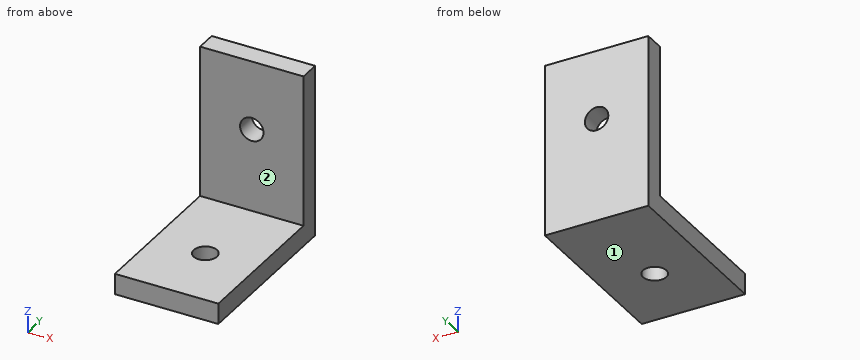
```python
from build123d import *

# Parameters (mm, degrees)
CROQUIS1_W           = 15
CROQUIS1_H           = 25
ALA_HORIZONTAL_DEPTH = 3
ALA_VERTICAL_START   = -3
CROQUIS2_W           = 15
CROQUIS2_H           = 25
ALA_VERTICAL_DEPTH   = 3
CROQUIS3_R           = 1.7
BARRENO_M3_H_DEPTH   = 3
BARRENO_M3_V_START   = -3
CROQUIS4_R           = 1.7
BARRENO_M3_V_DEPTH   = 3


with BuildPart() as part:
    # Croquis1 → Ala_horizontal (new body)
    with BuildSketch(Plane.XY):
        with Locations((0, -12.5)):
            Rectangle(CROQUIS1_W, CROQUIS1_H)
    extrude(amount=ALA_HORIZONTAL_DEPTH)

    # Croquis2 → Ala_vertical (add)
    with BuildSketch(Plane(origin=(0, 0, 0), x_dir=(1, 0, 0), z_dir=(0, 1, 0)).offset(ALA_VERTICAL_START)):
        with Locations((0, -12.5)):
            Rectangle(CROQUIS2_W, CROQUIS2_H)
    extrude(amount=ALA_VERTICAL_DEPTH)

    # Croquis3 → Barreno_M3_h (cut)
    with BuildSketch(Plane.XY):
        with Locations((0, -15)):
            Circle(CROQUIS3_R)
    extrude(amount=BARRENO_M3_H_DEPTH, mode=Mode.SUBTRACT)

    # Croquis4 → Barreno_M3_v (cut)
    with BuildSketch(Plane(origin=(0, 0, 0), x_dir=(1, 0, 0), z_dir=(0, 1, 0)).offset(BARRENO_M3_V_START)):
        with Locations(Location((0, -15, 0), (0, 0, 270))):
            Circle(CROQUIS4_R)
    extrude(amount=BARRENO_M3_V_DEPTH, mode=Mode.SUBTRACT)


solid = part.part
```
Build history of the part. All positions in model axes, mm. Face numbers are marked on the shaded views. A direction names the side the tool comes from. Coordinates: 2 decimals unless noted, no trailing zeros. Order: outer loops, then holes, each group sorted by start corner. A loop starts at its lowest first (then second) coordinate and runs counter-clockwise, first axis right, second up. Notation, with made-up numbers: (37.5, -10) -> (83.5, -10) arc R16 ccw to (83.5, 19) -> close; hole circle Ø6 at (65, 20.5). An arc over 180 degrees is marked (long way). Answer in a Markdown table with one row per item. Add a question column.
Q1. Band-saw the part on A-A, the plane x = 0. List the corners of the cut face in (y, z).
Q2. Which spindle directions (+Z, -Z, +X, -X, +Y, -Y) get a long thin tool onto all of the face, cutting with end or side? Do the marked faces 1 and 2. Say none if no direction does.
Q3. Wall check: line 1 along Y through (x, z) = (0, 1.05); line 2 along X through (y, z) = (-1.85, 15); line 3 along Y through (x, z) = (-5.75, 13.5). Give the ranges that are in metal, low to high. Write a range as [from, to].
Q4. Band-saw the part on D-D, the plane x = 2.5. List the corners of the cut face in (y, z).
Q5. Drop a flat-ended pin along its axis: pin 1 (8 mm diameter, centred on x = 3.5, z = 22, fed in from -Y). Give the stop position or say it passes through.
Q6. Band-saw the part on C-C, the plane z = 15. List the corners of the cut face in (x, y), then the cut area to 3 significant figures.
Q7. Band-saw the part on B-B, the plane y = -15. List the corners of the cut face in (x, z).
Answers follow:
| question | item | result |
|---|---|---|
| 1 | outline | (-25, 0) -> (-16.7, 0) -> (-16.7, 3) -> (-25, 3) -> close; (-13.3, 0) -> (0, 0) -> (0, 13.3) -> (-3, 13.3) -> (-3, 3) -> (-13.3, 3) -> close; (-3, 16.7) -> (0, 16.7) -> (0, 25) -> (-3, 25) -> close |
| 2 | face 1 | -Z, +X, -X, +Y, -Y |
| 2 | face 2 | +Z, +X, -X, -Y |
| 3 | line 1 | [-25, -16.7], [-13.3, 0] |
| 3 | line 2 | [-7.5, -1.7], [1.7, 7.5] |
| 3 | line 3 | [-3, 0] |
| 4 | outline | (-25, 0) -> (0, 0) -> (0, 25) -> (-3, 25) -> (-3, 3) -> (-25, 3) -> close |
| 5 | pin 1 | y = -3 |
| 6 | outline | (-7.5, -3) -> (-1.7, -3) -> (-1.7, 0) -> (-7.5, 0) -> close; (1.7, -3) -> (7.5, -3) -> (7.5, 0) -> (1.7, 0) -> close |
| 6 | area | 34.8 mm^2 |
| 7 | outline | (-7.5, 0) -> (-1.7, 0) -> (-1.7, 3) -> (-7.5, 3) -> close; (1.7, 0) -> (7.5, 0) -> (7.5, 3) -> (1.7, 3) -> close |
